from build123d import *

# Parameters (mm, degrees)
ESQUISSE1_R        = 5.5
BOSS_EXTRU_1_DEPTH = 5
ESQUISSE2_W        = 10
ESQUISSE2_H        = 38
ESQUISSE2_W_2      = 25
ESQUISSE2_H_2      = 10
BOSS_EXTRU_2_DEPTH = 6
D_POUILLE3_ANGLE   = 10
BOSS_EXTRU_3_DEPTH = 30
CHANFREIN3_SIZE    = 5


with BuildPart() as part:
    # Esquisse1 → Boss.-Extru.1 (new body)
    with BuildSketch(Plane.XY):
        Polygon((0, 0), (0, 90), (45, 90), (122, 45), (122, 0), align=None)
        with Locations((22.5, 75)):
            Circle(ESQUISSE1_R, mode=Mode.SUBTRACT)
        with Locations((22.5, 15)):
            Circle(ESQUISSE1_R, mode=Mode.SUBTRACT)
        with Locations((107, 22.5)):
            Circle(ESQUISSE1_R, mode=Mode.SUBTRACT)
        with Locations((60, 22.5)):
            Circle(ESQUISSE1_R, mode=Mode.SUBTRACT)
    extrude(amount=BOSS_EXTRU_1_DEPTH)

    # Esquisse2 → Boss.-Extru.2 (add)
    with BuildSketch(Plane.XY):
        with Locations((22.5, 45)):
            Rectangle(ESQUISSE2_W, ESQUISSE2_H)
        with Locations((83.5, 22.5)):
            Rectangle(ESQUISSE2_W_2, ESQUISSE2_H_2)
    extrude(amount=-BOSS_EXTRU_2_DEPTH)

    # Dépouille3
    d_pouille3_faces = [part.faces().sort_by_distance(p)[0] for p in [
        (83.5, 27.5, -3),
        (96, 22.5, -3),
        (71, 22.5, -3),
        (83.5, 17.5, -3),
        (22.5, 26, -3),
        (27.5, 45, -3),
        (22.5, 64, -3),
        (17.5, 45, -3),
    ]]
    draft(d_pouille3_faces, Plane(origin=(0, 0, 0), x_dir=(-1, 0, 0), z_dir=(0, 0, -1)), D_POUILLE3_ANGLE)

    # Esquisse3 → Boss.-Extru.3 (add)
    with BuildSketch(Plane(origin=(0, 0, 0), x_dir=(-1, 0, 0), z_dir=(0, 0, -1))):
        Polygon((-122, 45), (-45, 45), (-45, 90), align=None)
    extrude(amount=BOSS_EXTRU_3_DEPTH)

    # Chanfrein3
    chanfrein3_edges = [part.edges().sort_by_distance(p)[0] for p in [
        (45, 45, -15),
    ]]
    chamfer(chanfrein3_edges, length=CHANFREIN3_SIZE)


solid = part.part
Read the model definition and answer for the solid it produces. Units are mm, in the model's axes. A direction names the side the tool comes from. Round coordinates to 2 decimals unless told otherwise and drop trailing zeros. Write each loop counter-clockwise with the first axis right and the second up, starting at its lowest first coordinate (ties: lowest second). Pieces come first, ordered by that corner, then holes. Notation, with made-up numbers: (-36, 29) - (0, 29) arc R20 cw to (0, 55) - close; hole circle Ø4 at (28, 73.5). An arc over 180 degrees is marked (long way). Use a Markdown table: item, result.
(1) The part is cut by section B-B (x = 22.5). Write down the section's boundary in (y, z).
Reported:
| item | result |
|---|---|
| outline | (0, 0) - (9.5, 0) - (9.5, 5) - (0, 5) - close; (20.5, 0) - (26, 0) - (27.06, -6) - (62.94, -6) - (64, 0) - (69.5, 0) - (69.5, 5) - (20.5, 5) - close; (80.5, 0) - (90, 0) - (90, 5) - (80.5, 5) - close |
(2) Each of these flat-tipped pins is pushed along its axis until it touches: pin 1 Ø5 at (x, z) = (104.5, -13.5) entering from -Y; pin 2 Ø10 at (x, z) = (91, -8) entering from +Y; pin 3 Ø1 at (y, z) = (48, 1) entering from +X; pin 4 Ø6.5 at (x, y) = (60, 22.5) entering from -Z. Where does it stop, or does it pass through?
Reported:
| item | result |
|---|---|
| pin 1 | y = 45 |
| pin 2 | y = 66.04 |
| pin 3 | x = 117.72 |
| pin 4 | through |
(3) The part is cut by section D-D (z = -2). Write down the section's boundary in (x, y), then the cut area to 3 significant figures.
Reported:
| item | result |
|---|---|
| outline | (17.85, 26.35) - (27.15, 26.35) - (27.15, 63.65) - (17.85, 63.65) - close; (45, 50) - (50, 45) - (122, 45) - (45, 90) - close; (71.35, 17.85) - (95.65, 17.85) - (95.65, 27.15) - (71.35, 27.15) - close |
| area | 2,290 mm2 |
(4) The part is cut by section C-C (x = 105.5). Write down the section's boundary in (y, z).
Reported:
| item | result |
|---|---|
| outline | (0, 0) - (17.21, 0) - (17.21, 5) - (0, 5) - close; (27.79, 0) - (45, 0) - (45, -30) - (54.64, -30) - (54.64, 5) - (27.79, 5) - close |
(5) Which of the six approach directions +Z, -Z, +X, -X, +Y, -Y give full straight-line access (tool end or side, diameter ignored) to faces 4 (the flat face through (22, 45, -6)), 5 (the flat face through (83.32, 26.98, -2.96)), 6 (the flat face through (22.43, 26.52, -2.96)), 7 (the flat face through (47, 48, -15)), 8 (the flat face through (83, 23, -6))?
Reported:
| item | result |
|---|---|
| face 4 | -Z, -X, +Y, -Y |
| face 5 | -Z, +X |
| face 6 | -Z, -X, -Y |
| face 7 | -Z, -Y |
| face 8 | -Z, +X, -X, -Y |
(6) The mould has two halves that part along X. Classify faces 1 (the flat face through (95.48, 22.43, -2.96)), 2 (the flat face through (22, 90, 2)), 3 (the flat face through (26.98, 44.73, -2.96)): released by +X, released by -X, zero draft, split by the parting line, or undercut.
Reported:
| item | result |
|---|---|
| face 1 | released by +X |
| face 2 | zero draft |
| face 3 | undercut |
(7) The part is cut by section A-A (y = 22.5). Write down the section's boundary in (x, z).
Reported:
| item | result |
|---|---|
| outline | (0, 0) - (54.5, 0) - (54.5, 5) - (0, 5) - close; (65.5, 0) - (71, 0) - (72.06, -6) - (94.94, -6) - (96, 0) - (101.5, 0) - (101.5, 5) - (65.5, 5) - close; (112.5, 0) - (122, 0) - (122, 5) - (112.5, 5) - close |
(8) Straight lines are drawn through the part: line 1 along Y through (x, z) = (22, 3); line 2 along X through (y, z) = (22, 2); line 3 along Z through (x, y) = (115, 24.5). For each, find the intervals that lie inside material, in ascending order. Write a range as [from, to].
Reported:
| item | result |
|---|---|
| line 1 | [0, 9.52], [20.48, 69.52], [80.48, 90] |
| line 2 | [0, 54.52], [65.48, 101.52], [112.48, 122] |
| line 3 | [0, 5] |
